Build history of the part. All positions in model axes, mm. Face numbers are marked on the shaded views. A direction names the side the tool comes from. Coordinates: 2 decimals unless noted, no trailing zeros. Order: outer loops, then holes, each group sorted by start corner. A loop starts at its lowest first (then second) coordinate and runs counter-clockwise, first axis right, second up. Notation, with made-up numbers: (-4, 79) - (8, 79) arc R20 cw to (8, 105) - close; hole circle Ø8 at (-9, 13.5). An arc over 180 degrees is marked (long way). Write each question's results on one line, items separated by ' | '.
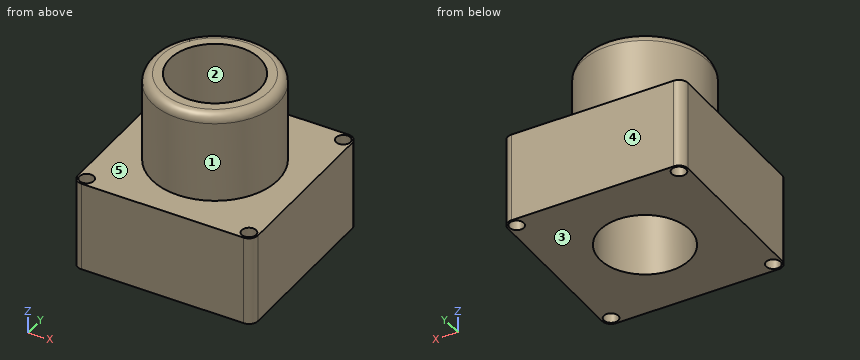
Autodesk Inventor part; units mm, degrees
ref_plane "YZ Plane" through (0, 0, 0) normal (1, 0, 0) x (0, 1, 0)
ref_plane "XZ Plane" through (0, 0, 0) normal (0, 1, 0) x (-1, 0, 0)
ref_plane "XY Plane" through (0, 0, 0) normal (0, 0, 1) x (1, 0, 0)
sketch "Sketch1" plane through (0, 0, 0) normal (0, 0, 1) x (1, 0, 0)
  line L0 (0, 0) -> (100, 0)
  line L1 (100, 0) -> (100, 100)
  line L2 (100, 100) -> (0, 100)
  line L3 (0, 100) -> (0, 0)
  dimension "d0" = 100
  dimension "d1" = 100
extrude "Extrusion1" add sketch "Sketch1" along normal blind 50
sketch "Sketch2" plane through (0, 0, 50) normal (0, 0, 1) x (1, 0, 0)
  line L0 (100, 100) -> (0, 100)
  line L1 (50, 100) -> (50, 0)
  line L2 (0, 100) -> (0, 0)
  line L3 (0, 50) -> (100, 50)
  circle A0 centre (50, 50) radius 35
  dimension "d4" = 70
extrude "Extrusion2" add sketch "Sketch2" along normal blind 50 contours A0 L3 L1 | L1 L3 A0 | L3 A0 L1 | L1 A0 L3
fillet "Fillet1" radius 5 4 edges at (100, 100, 25) (0, 100, 25) (0, 0, 25) (100, 0, 25)
sketch "Sketch3" plane through (50, 50, 100) normal (0, 0, 1) x (1, 0, 0)
  circle A0 centre (0, 0) radius 25
  point P0 (-50, -50)
  dimension "d8" = 50
extrude "Extrusion3" cut sketch "Sketch3" against normal blind 100
fillet "Fillet2" radius 5 1 edges at (15, 50, 100)
sketch "Sketch4" plane through (0, 0, 50) normal (0, 0, 1) x (1, 0, 0)
  arc A0 (0, 5) -> (5, 0) centre (5, 5) ccw construction
  circle A1 centre (5, 5) radius 4
  arc A2 (95, 0) -> (100, 5) centre (95, 5) ccw
  circle A3 centre (95, 5) radius 4
  arc A4 (100, 95) -> (95, 100) centre (95, 95) ccw
  circle A5 centre (95, 95) radius 4
  arc A6 (5, 100) -> (0, 95) centre (5, 95) ccw
  circle A7 centre (5, 95) radius 4
  point P0 (0, 0)
extrude "Extrusion4" cut sketch "Sketch4" against normal blind 100
thread "Thread1"
properties part number "Tarea1"
1. Tool access for the marked faces 4 and 5: list every direction of +Z, -Z, +X, -X, +Y, -Y with a clear straight run to the whole face (end or side of a thin tool).
Solved:
face 4: +Z, -Z, +X, -X, +Y | face 5: +Z
2. Drop flat-ended pins along their axis: pin 1 Ø6 at (x, z) = (75, 63) entering from +Y; pin 2 Ø10.5 at (x, y) = (5, 5) entering from +Z; pin 3 Ø1 at (x, z) = (77, 58) entering from -Y. Give the stop position or say it passes through.
Solved:
pin 1: stops at y = 77.22 | pin 2: stops at z = 50 | pin 3: stops at y = 27.14
3. Probe line 1 (Y direction, x = 95, z = 35.5); line 2 (Y direction, x = 50, z = 22); line 3 (Y direction, x = 96, z = 12). List the from-to ranges inside material, lowest first.
Solved:
line 1: y = 0 to 1, 9 to 91, 99 to 100 | line 2: y = 0 to 25, 75 to 100 | line 3: y = 0.1 to 1.13, 8.87 to 91.13, 98.87 to 99.9
4. Band-saw the part on D-D on z = 93. Give the cut face in (x, y).
Solved:
outline: circle Ø70 at (50, 50); hole circle Ø50 at (50, 50)
5. Two-plate mould, pull along X, no slides. Class the marked faces 1, 2 and 3: +X half, -X half, draft (parallel to the pull), parting line (faces both ways), or undercut.
Solved:
face 1: parting line | face 2: undercut | face 3: draft
6. Band-saw the part on A-A on x = 50. Give the cut face in (y, z), then the cut area to 3 significant figures.
Solved:
outline: (0, 0) - (25, 0) - (25, 100) - (20, 100) arc R5 ccw to (15, 95) - (15, 50) - (0, 50) - close; (75, 0) - (100, 0) - (100, 50) - (85, 50) - (85, 95) arc R5 ccw to (80, 100) - (75, 100) - close | area: 3,490 mm2
7. Band-saw the part on C-C on y = 92.5. Give the cut face in (x, z), then the cut area to 3 significant figures.
Solved:
outline: (0, 0) - (1.88, 0) - (1.88, 50) - (0, 50) - close; (8.12, 0) - (91.88, 0) - (91.88, 50) - (8.12, 50) - close; (98.12, 0) - (100, 0) - (100, 50) - (98.12, 50) - close | area: 4,380 mm2
8. Band-saw the part on B-B on z = 9. Give the cut face in (x, y).
Solved:
outline: (0, 5) arc R5 ccw to (5, 0) - (95, 0) arc R5 ccw to (100, 5) - (100, 95) arc R5 ccw to (95, 100) - (5, 100) arc R5 ccw to (0, 95) - close; hole circle Ø8 at (5, 5); hole circle Ø8 at (5, 95); hole circle Ø50 at (50, 50); hole circle Ø8 at (95, 5); hole circle Ø8 at (95, 95)
